Read the model definition and answer for the solid it produces. Units are mm, in the model's axes. A direction names the side the tool comes from. Coordinates: 2 decimals unless noted, no trailing zeros. Loops run counter-clockwise (first coordinate to the right, second up) from the corner with the lowest first, then second, coordinate; pieces in that order, holes last. Notation, with made-up numbers: (44, 17) - (63, 17) arc R16 ccw to (63, 39) - close; hole circle Ø1 at (-2, 4.25). An arc over 180 degrees is marked (long way). Use CSV: the item, a comma, the result in double quotes.
```python
from build123d import *

# Parameters (mm, degrees)
SKETCH1_R                      = 25
BOSS_EXTRUDE1_DEPTH            = 25
CUT_EXTRUDE1_DEPTH             = 50
CUT_EXTRUDE2_REACH             = 138.931
SKETCH3_W                      = 6.698729811
SKETCH3_H                      = 50
CUT_EXTRUDE2_DIRECTION_2_REACH = 138.931


with BuildPart() as part:
    # Sketch1 → Boss-Extrude1 (new, symmetric)
    with BuildSketch(Plane.XY):
        with BuildLine():
            Line((-75, 50), (75, 50))
            ThreePointArc((75, 50), (125, 0), (75, -50))
            Line((75, -50), (-75, -50))
            ThreePointArc((-75, -50), (-125, 0), (-75, 50))
        make_face()
        with Locations((-75, 0)):
            Circle(SKETCH1_R, mode=Mode.SUBTRACT)
    extrude(amount=BOSS_EXTRUDE1_DEPTH, both=True)

    # Sketch2 → Cut-Extrude1 (cut)
    with BuildSketch(Plane(origin=(75, 0, 0), x_dir=(0, 0, -1), z_dir=(1, 0, 0))):
        with BuildLine():
            Line((25, 50), (-25, 50))
            Line((-25, 50), (-25, -5.1e-08))
            ThreePointArc((-25, -5.1e-08), (-2.6e-08, 25), (25, 0))
            Line((25, 0), (25, 50))
        make_face()
        with BuildLine():
            ThreePointArc((25, 0), (2.6e-08, -25), (-25, -5.1e-08))
            Line((-25, -5.1e-08), (-25, -50))
            Line((-25, -50), (25, -50))
            Line((25, -50), (25, 0))
        make_face()
    extrude(amount=CUT_EXTRUDE1_DEPTH, mode=Mode.SUBTRACT)

    # Sketch3 → Cut-Extrude2 (cut, up to next)
    with BuildSketch(Plane.XY, mode=Mode.PRIVATE) as cut_extrude2_sk1:
        with Locations((121.650635095, 0)):
            Rectangle(SKETCH3_W, SKETCH3_H)
    cut_extrude2_tool1 = extrude(cut_extrude2_sk1.sketch, amount=-CUT_EXTRUDE2_REACH, mode=Mode.PRIVATE) & part.part
    add(cut_extrude2_tool1.solids().sort_by_distance((121.650635, 0, 0))[0], mode=Mode.SUBTRACT)

    # Sketch3 → Cut-Extrude2 direction 2 (cut, up to next)
    with BuildSketch(Plane.XY, mode=Mode.PRIVATE) as cut_extrude2_direction_2_sk1:
        with Locations((121.650635095, 0)):
            Rectangle(SKETCH3_W, SKETCH3_H)
    cut_extrude2_direction_2_tool1 = extrude(cut_extrude2_direction_2_sk1.sketch, amount=CUT_EXTRUDE2_DIRECTION_2_REACH, mode=Mode.PRIVATE) & part.part
    add(cut_extrude2_direction_2_tool1.solids().sort_by_distance((121.650635, 0, 0))[0], mode=Mode.SUBTRACT)


solid = part.part
```
Q1. The part is cut by section D-D on z = -17. Determine the outline of the cut face in (x, y), and give its area (3 significant figures).
Reported:
outline,"(-75, -50) - (75, -50) - (75, -18.33) - (118.3, -18.33) - (118.3, 18.33) - (75, 18.33) - (75, 50) - (-75, 50) arc R50 ccw to start; hole circle Ø50 at (-75, 0)"
area,"18,600 mm²"
Q2. Given P1, Ø8, axis at y = 26.5, z = 18, coming from the +X side; P2, Ø8, axis at y = 6, z = 10, coming from the -X side; P3, Ø1, axis at y = 36, z = 7, coming from the -X side, each flat-ended and moving along its own axis, determine where each tip first touches the part or whether it passes through.
Reported:
P1,"stops at x = 75"
P2,"stops at x = -124.96"
P3,"stops at x = -110.21"
Q3. The part is cut by section C-C on x = -80. Determine the outline of the cut face in (y, z).
Reported:
outline,"(-49.75, -25) - (-24.49, -25) - (-24.49, 25) - (-49.75, 25) - close; (24.49, -25) - (49.75, -25) - (49.75, 25) - (24.49, 25) - close"
Q4. The part is cut by section B-B on y = -5.5. Determine the outline of the cut face in (x, z).
Reported:
outline,"(-124.7, -25) - (-99.39, -25) - (-99.39, 25) - (-124.7, 25) - close; (-50.61, -25) - (75, -25) - (75, -24.39) - (118.3, -24.39) - (118.3, 24.39) - (75, 24.39) - (75, 25) - (-50.61, 25) - close"
Q5. The part is cut by section A-A on z = 0. Determine the outline of the cut face in (x, y), and give its area (3 significant figures).
Reported:
outline,"(-75, -50) - (75, -50) - (75, -25) - (118.3, -25) - (118.3, 25) - (75, 25) - (75, 50) - (-75, 50) arc R50 ccw to start; hole circle Ø50 at (-75, 0)"
area,"19,100 mm²"
Q6. A tool of negligible diameter and unlimited length cuts with its end or side. For faces 1 (the face through (96.348, -7.509, -23.846)), 2 (the face through (75, -36, 0)), 3 (the face through (-1, 50, 0)), from which of +Z, -Z, +X, -X, +Y, -Y can it reach the whole face along a straight path? Write none if from no direction.
Reported:
face 1,"+X"
face 2,"+X, -Y"
face 3,"+Z, -Z, +X, -X, +Y"
Q7. For a pull along X with two mould halves and no side action, classify faces 4 (the face through (118.301, 0, 0)), 5 (the face through (-95, -15, 0)), 6 (the face through (-124.988, -1.099, 0.35)), 7 (the face through (-24, 1, -25)) as +X half, -X half, draft (parallel to the pull), parting line (faces both ways), or undercut.
Reported:
face 4,"+X half"
face 5,"undercut"
face 6,"-X half"
face 7,"draft"
Q8. Find the intervals of material crossed by probe 1 along Y at (x, z) = (-75, 3); probe 2 along X at (y, z) = (-21, -1.5); probe 3 along X at (y, z) = (3.5, 23), in increasing order. Write a range as [from, to].
Reported:
probe 1,"y = [-50, -25], [25, 50]"
probe 2,"x = [-120.38, -88.56], [-61.44, 118.3]"
probe 3,"x = [-124.88, -99.75], [-50.25, 118.3]"
